```python
from build123d import *

# Parameters (mm, degrees)
F2_W      = 5
F2_H      = 5
F4_DEPTH  = 2.13
F5_DEPTH  = 2.13
F6_W      = 33
F6_H      = 12
F7_DEPTH  = 1
F9_DEPTH  = 2.13
F10_W     = 3
F10_H     = 10
F11_DEPTH = 1.5


with BuildPart() as f4:
    # F2 (on Top) → F4 (new body)
    with BuildSketch(Plane.XY):
        Rectangle(F2_W, F2_H)
    extrude(amount=F4_DEPTH)



with BuildPart() as f5:
    # F3 (on face) → F5 (new body)
    with BuildSketch(Plane.XY):
        with BuildLine():
            ThreePointArc((5.905, 0), (4.6210978184, 1.800906022), (2.5, 1.1743189516))
            Line((2.5, 1.1743189516), (2.5, -1.1743189516))
            ThreePointArc((2.5, -1.1743189516), (4.6210978184, -1.800906022), (5.905, 0))
        make_face()
    extrude(amount=F5_DEPTH)


with BuildPart() as f7:
    # F6 (on face) → F7 (new body)
    with BuildSketch(Plane.XY):
        Rectangle(F6_W, F6_H)
    extrude(amount=-F7_DEPTH)


with BuildPart() as f4_1:
    add(f4.part)

    add(f5.part)  # F9 merges F5

    add(f7.part)  # F9 merges F7
    # F8 (on face) → F9 (join, through all)
    with BuildSketch(Plane.XY):
        with BuildLine():
            Line((2, 3.7145), (-2, 3.7145))
            ThreePointArc((-2, 3.7145), (-3.2123345763, 3.2123345763), (-3.7145, 2))
            Line((-3.7145, 2), (-3.7145, -2))
            ThreePointArc((-3.7145, -2), (-3.2123345763, -3.2123345763), (-2, -3.7145))
            Line((-2, -3.7145), (2, -3.7145))
            ThreePointArc((2, -3.7145), (3.2123345763, -3.2123345763), (3.7145, -2))
            Line((3.7145, -2), (3.7145, 2))
            ThreePointArc((3.7145, 2), (3.2123345763, 3.2123345763), (2, 3.7145))
        make_face()
    extrude(amount=F9_DEPTH)

    # F10 (on face) → F11 (join)
    with BuildSketch(Plane.XY):
        with Locations((-15, 0)):
            Rectangle(F10_W, F10_H)
        with Locations((15, 0)):
            Rectangle(F10_W, F10_H)
    extrude(amount=F11_DEPTH)


solid = f4_1.part
```
CAD build for the part. Positions are in the model's coordinates, mm. A direction names the side the tool comes from. Give positions to 0.01 mm unless a question says otherwise; leave off trailing zeros. Write each loop counter-clockwise with the first axis right and the second up, starting at its lowest first coordinate (ties: lowest second). Pieces come first, ordered by that corner, then holes. Notation, with made-up numbers: M 16.25,62 L 37.25,62 A13 cw 37.25,77 Z; hole C 32.5,-21.5 d9. An arc over 180 degrees is marked long. Return JSON: item names as keys, results as strings. Group by question number.
(1) Drill centre lines: L1, parallel to X at y = -2.5, z = 0.85; L2, parallel to X at y = -0.25, z = 0.2; L3, parallel to Z at x = -4.5, y = 1.5. Where is each one in solid material? Low to high. Write a range as [from, to].
(2) Band-saw the part on B-B (y = 4). Give the cut face in (x, z), and give its area (3 significant figures).
(3) Mould opens along X. For faces 6 (the face through (-4, 0, 0)), 7 (the face through (-16.5, 0, 0)), 8 (the face through (-15, -5, 1)), 9 (the face through (3.226, 3.199, 1.05)) say: pulls with the +X half, pulls with the -X half, needs draft (parallel to the pull), parting line crosses it, or undercut.
(4) 3-axis set-ups, long thin cutter, end or side, ignore diameter. For faces 1 (the face through (-15, 5, 1)), 2 (the face through (-15, 0, 1.5)), 3 (the face through (-13.5, 0, 1)), 4 (the face through (-3.199, 3.226, 1.05)), 5 (the face through (15, 0, 1.5)): which of +Z, -Z, +X, -X, +Y, -Y reach the whole face in a straight line?
(5) Band-saw the part on D-D (x = -10.5). Give the cut face in (y, z).
(6) Band-saw the part on C-C (y = -1.25). Give the cut face in (x, z).
(7) Band-saw the part on A-A (x = 4). Give the cut face in (y, z) (3 decimals), and give its area (3 significant figures).
(8) Flat gauge pins, fed straight in: pin 1 Ø1.6 at (x, z) = (-15.5, 0.5) entering from +Y; pin 2 Ø1.5 at (x, z) = (1.5, 2) entering from -Y; pin 3 Ø3.5 at (x, y) = (-15.5, 1.5) entering from +Z; pin 4 Ø0.6 at (x, z) = (0.5, 0.5) entering from +Y. Where does each tip first touch, or does it go through?
Entries:
{
 "1": {"L1": "x = [-16.5, -13.5], [-3.64, 3.64], [13.5, 16.5]", "L2": "x = [-16.5, -13.5], [-3.71, 5.89], [13.5, 16.5]", "L3": "z = [-1, 0]"},
 "2": {"outline": "M -16.5,-1 L 16.5,-1 L 16.5,1.5 L 13.5,1.5 L 13.5,0 L -13.5,0 L -13.5,1.5 L -16.5,1.5 Z", "area": "42.0 mm^2"},
 "3": {"face 6": "undercut", "face 7": "pulls with the -X half", "face 8": "needs draft", "face 9": "undercut"},
 "4": {"face 1": "+Z, +X, -X, +Y", "face 2": "+Z, -X, +Y, -Y", "face 3": "+Z, +Y, -Y", "face 4": "+Z, +Y", "face 5": "+Z, +X, +Y, -Y"},
 "5": {"outline": "M -6,-1 L 6,-1 L 6,0 L -6,0 Z"},
 "6": {"outline": "M -16.5,-1 L 16.5,-1 L 16.5,1.5 L 13.5,1.5 L 13.5,0 L 5.44,0 L 5.44,2.13 L -3.71,2.13 L -3.71,0 L -13.5,0 L -13.5,1.5 L -16.5,1.5 Z"},
 "7": {"outline": "M -6,-1 L 6,-1 L 6,0 L 1.905,0 L 1.905,2.13 L -1.905,2.13 L -1.905,0 L -6,0 Z", "area": "20.1 mm^2"},
 "8": {"pin 1": "stops at y = 6", "pin 2": "stops at y = -3.71", "pin 3": "stops at z = 1.5", "pin 4": "stops at y = 3.71"}
}
